Print and shaded views of the part. All mm, measured from the part's lowest x, y and z. A direction names the side the tool comes from. Round coordinates to 2 decimals unless told otherwise and drop trailing zeros. Order: outer loops, then holes, each group sorted by start corner. A loop starts at its lowest first (then second) coordinate and runs counter-clockwise, first axis right, second up. Notation, with made-up numbers: (66.5, 53.25) - (91.5, 53.25) arc R26 ccw to (91.5, 90.25) - close; hole circle Ø3 at (-11.5, 31.25). An arc over 180 degrees is marked (long way). Write item = value, one per line.
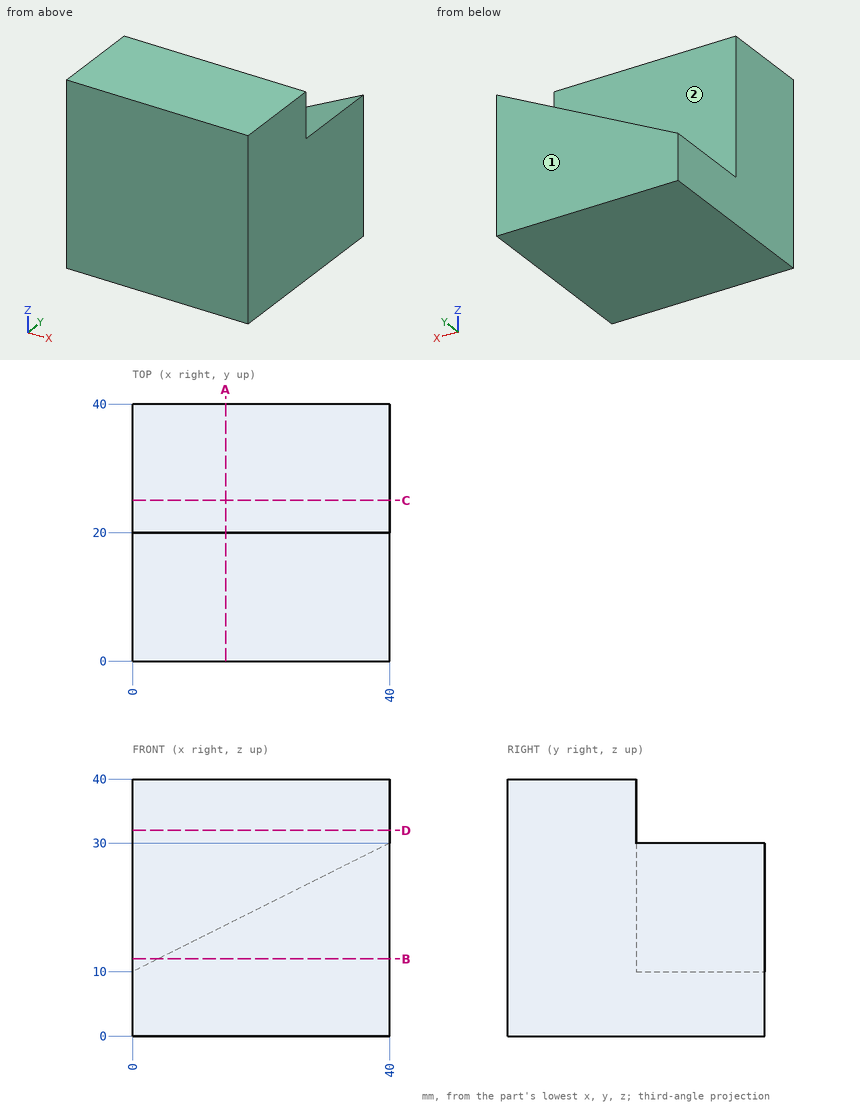
(1) Band-saw the part on A-A on x = 14.5. List the corners of the cut face in (y, z).
Solved:
outline = (0, 0) - (40, 0) - (40, 17.25) - (20, 17.25) - (20, 40) - (0, 40) - close
(2) Band-saw the part on C-C on y = 25. List the corners of the cut face in (x, z), plus the area to 3 significant figures.
Solved:
outline = (0, 0) - (40, 0) - (40, 30) - (0, 10) - close
area = 800 mm²
(3) Band-saw the part on D-D on z = 32. List the corners of the cut face in (x, y), plus the area to 3 significant figures.
Solved:
outline = (0, 0) - (40, 0) - (40, 20) - (0, 20) - close
area = 800 mm²
(4) Band-saw the part on B-B on z = 12. List the corners of the cut face in (x, y), plus the area to 3 significant figures.
Solved:
outline = (0, 0) - (40, 0) - (40, 40) - (4, 40) - (4, 20) - (0, 20) - close
area = 1,520 mm²
(5) Tool access for the marked faces 1 and 2: list every direction of +Z, -Z, +X, -X, +Y, -Y with a clear straight run to the whole face (end or side of a thin tool).
Solved:
face_1 = +Z, -Z, +X, -X, +Y
face_2 = +Z, -X, +Y
(6) Probe line 1 along Y through (x, z) = (14, 20); line 2 along Z through (x, y) = (31, 31); line 3 along Z through (x, y) = (21.5, 24.5). List the from-to ranges inside material, lowest first.
Solved:
line_1 = 0 to 20
line_2 = 0 to 25.5
line_3 = 0 to 20.75
(7) Drop flat-ended pins along their axis: pin 1 (4 mm diameter, centred on y = 23.5, z = 34, fed in from -X); pin 2 (2 mm diameter, centred on y = 32, z = 15.5, fed in from -X); pin 3 (2 mm diameter, centred on x = 4.5, z = 17, fed in from +Y). Give the stop position or say it passes through.
Solved:
pin_1 = through
pin_2 = 9
pin_3 = 20
